Verification items for the finished model (mm, model axes). A direction names the side the tool comes from. Round coordinates to 2 decimals unless told otherwise and drop trailing zeros. Write each loop counter-clockwise with the first axis right and the second up, starting at its lowest first coordinate (ties: lowest second). Pieces come first, ordered by that corner, then holes. Notation, with made-up numbers: (18, 40) - (56, 40) arc R18 ccw to (56, 49) - close; hole circle Ø3 at (57.25, 68.25). An arc over 180 degrees is marked (long way). Answer as a JSON object with one key per item and string values.
Autodesk Inventor part; units mm, degrees
ref_plane "cut1_XY" through (13.4874, 7.874, 0) normal (1, 0, 0) x (0, 0, -1)
ref_plane "cut1_YZ" through (13.4874, 7.874, 0) normal (0, 0, -1) x (0, 1, 0)
ref_plane "cut1_ZX" through (13.4874, 7.874, 0) normal (0, 1, 0) x (1, 0, 0)
sketch "Sketch_1" plane through (0, 0, 0) normal (0, 0, 1) x (1, 0, 0)
  line L0 (13.4874, 0) -> (0, 0)
  line L1 (0, 0) -> (0, 8.9091)
  line L2 (0, 8.9091) -> (0.762, 9.671)
  line L3 (0.762, 9.671) -> (4.0386, 9.671)
  line L4 (4.0386, 9.671) -> (4.8006, 8.9091)
  line L5 (4.8006, 8.9091) -> (5.5626, 8.9091)
  line L6 (5.5626, 8.9091) -> (5.5626, 10.2235)
  line L7 (5.5626, 10.2235) -> (13.4874, 10.2235)
  line L8 (13.4874, 10.2235) -> (13.4874, 0)
  line L9 (13.4874, 0) -> (0, 0)
revolve "Revolution1" add sketch "Sketch_1" angle 360 about axis through (13.4874, 0, 0) along (1, 0, 0)
sketch "Sketch_6" plane through (0, 0, 0) normal (0, 0, 1) x (1, 0, 0)
  line L0 (13.4874, 0) -> (0, 0)
  line L1 (0, 0) -> (0, 4.3688)
  line L2 (0, 4.3688) -> (-1.5889, 4.3688)
  line L3 (-1.5889, 4.3688) -> (12.8524, 4.8197)
  line L4 (12.8524, 4.8197) -> (13.4874, 5.4547)
  line L5 (13.4874, 5.4547) -> (13.4874, 0)
  line L6 (13.4874, 0) -> (0, 0)
revolve "Revolution2" cut sketch "Sketch_6" angle 360 about axis through (13.4874, 0, 0) along (1, 0, 0)
thread "Thread1"
sketch "Sketch_5" plane through (13.4874, 0, 0) normal (1, 0, 0) x (0, 0, -1)
  line L0 (-40.894, -20.447) -> (40.894, -20.447)
  line L1 (40.894, -20.447) -> (40.894, 20.447)
  line L2 (40.894, 20.447) -> (-40.894, 20.447)
  line L3 (-40.894, 20.447) -> (-40.894, -20.447)
  line L4 (-20.447, -7.874) -> (20.447, -7.874)
  line L5 (20.447, -7.874) -> (20.447, 7.874)
  line L6 (20.447, 7.874) -> (-20.447, 7.874)
  line L7 (-20.447, 7.874) -> (-20.447, -7.874)
extrude "Extrusion1" cut sketch "Sketch_5" against normal blind 4.7752
sketch "Sketch_24" plane through (0, 0, 0) normal (0, 0, 1) x (1, 0, 0)
  line L0 (5.5626, 0) -> (4.8006, 0)
  line L1 (4.6479, 10.2235) -> (4.6479, 10.1393)
  line L2 (4.6479, 10.1393) -> (5.4401, 9.3472)
  arc A0 (5.4401, 9.1676) -> (5.4401, 9.3472) centre (5.3503, 9.2574) ccw
  line L3 (5.4401, 9.1676) -> (5.1816, 8.9091)
  line L4 (5.1816, 8.9091) -> (4.8006, 8.9091)
  line L5 (4.8006, 8.9091) -> (4.8006, 8.655)
  line L6 (4.8006, 8.655) -> (5.5626, 8.655)
  line L7 (5.5626, 8.655) -> (5.5626, 9.512)
  line L8 (5.5626, 9.512) -> (4.8511, 10.2235)
  line L9 (4.8511, 10.2235) -> (4.6479, 10.2235)
revolve "Revolution3" add sketch "Sketch_24" angle 360 about axis through (5.5626, 0, 0) along (1, 0, 0)
ref_plane "cut1_XY" through (13.4874, 7.874, 0) normal (1, 0, 0) x (0, 0, -1)
ref_plane "cut1_YZ" through (13.4874, 7.874, 0) normal (0, 0, -1) x (0, 1, 0)
ref_plane "cut1_ZX" through (13.4874, 7.874, 0) normal (0, 1, 0) x (1, 0, 0)
ref_plane "cut2_XY" through (13.4874, -7.874, 0) normal (1, 0, 0) x (0, 0, -1)
ref_plane "cut2_YZ" through (13.4874, -7.874, 0) normal (0, 0, -1) x (0, 1, 0)
ref_plane "cut2_ZX" through (13.4874, -7.874, 0) normal (0, 1, 0) x (1, 0, 0)
ref_plane "cutf1_XY" through (13.4874, 0, 0) normal (0, 0, 1) x (1, 0, 0)
ref_plane "cutf1_YZ" through (13.4874, 0, 0) normal (1, 0, 0) x (0, 1, 0)
ref_plane "cutf1_ZX" through (13.4874, 0, 0) normal (0, 1, 0) x (0, 0, 1)
ref_plane "cutf2_XY" through (8.7122, 0, 0) normal (0, 0, 1) x (1, 0, 0)
ref_plane "cutf2_YZ" through (8.7122, 0, 0) normal (1, 0, 0) x (0, 1, 0)
ref_plane "cutf2_ZX" through (8.7122, 0, 0) normal (0, 1, 0) x (0, 0, 1)
ref_plane "lovra_XY" through (13.4874, 0, 0) normal (1, 0, 0) x (0, 1, 0)
ref_plane "lovra_YZ" through (13.4874, 0, 0) normal (0, 1, 0) x (0, 0, 1)
ref_plane "lovra_ZX" through (13.4874, 0, 0) normal (0, 0, 1) x (1, 0, 0)
ref_plane "lovra1_XY" through (8.7122, 0, 0) normal (1, 0, 0) x (0, 0, -1)
ref_plane "lovra1_YZ" through (8.7122, 0, 0) normal (0, 0, -1) x (0, 1, 0)
ref_plane "lovra1_ZX" through (8.7122, 0, 0) normal (0, 1, 0) x (1, 0, 0)
ref_plane "lovra2_XY" through (8.7122, 7.874, 0) normal (1, 0, 0) x (0, 0, -1)
ref_plane "lovra2_YZ" through (8.7122, 7.874, 0) normal (0, 0, -1) x (0, 1, 0)
ref_plane "lovra2_ZX" through (8.7122, 7.874, 0) normal (0, 1, 0) x (1, 0, 0)
ref_plane "lovra21_XY" through (0, 0, 5.2705) normal (1, 0, 0) x (0, 0, -1)
ref_plane "lovra21_YZ" through (0, 0, 5.2705) normal (0, 0, -1) x (0, 1, 0)
ref_plane "lovra21_ZX" through (0, 0, 5.2705) normal (0, 1, 0) x (1, 0, 0)
ref_plane "lovra22_XY" through (0, 0, -5.2705) normal (1, 0, 0) x (0, 0, -1)
ref_plane "lovra22_YZ" through (0, 0, -5.2705) normal (0, 0, -1) x (0, 1, 0)
ref_plane "lovra22_ZX" through (0, 0, -5.2705) normal (0, 1, 0) x (1, 0, 0)
ref_plane "lovra3_XY" through (8.7122, -7.874, 0) normal (1, 0, 0) x (0, 0, -1)
ref_plane "lovra3_YZ" through (8.7122, -7.874, 0) normal (0, 0, -1) x (0, 1, 0)
ref_plane "lovra3_ZX" through (8.7122, -7.874, 0) normal (0, 1, 0) x (1, 0, 0)
ref_plane "olen_XY" through (13.4874, 0, 0) normal (1, 0, 0) x (0, 0, -1)
ref_plane "olen_YZ" through (13.4874, 0, 0) normal (0, 0, -1) x (0, 1, 0)
ref_plane "olen_ZX" through (13.4874, 0, 0) normal (0, 1, 0) x (1, 0, 0)
ref_plane "to_mounting_bracket_XY" through (24.6126, 0, 0) normal (1, 0, 0) x (0, 0, -1)
ref_plane "to_mounting_bracket_YZ" through (24.6126, 0, 0) normal (0, 0, -1) x (0, 1, 0)
ref_plane "to_mounting_bracket_ZX" through (24.6126, 0, 0) normal (0, 1, 0) x (1, 0, 0)
ref_plane "to_nut_XY" through (0, 0, 0) normal (1, 0, 0) x (0, 0, -1)
ref_plane "to_nut_YZ" through (0, 0, 0) normal (0, 0, -1) x (0, 1, 0)
ref_plane "to_nut_ZX" through (0, 0, 0) normal (0, 1, 0) x (1, 0, 0)
ref_plane "to_pin_XY" through (33.3248, 0, 0) normal (0, 1, 0) x (1, 0, 0)
ref_plane "to_pin_YZ" through (33.3248, 0, 0) normal (1, 0, 0) x (0, 0, -1)
ref_plane "to_pin_ZX" through (33.3248, 0, 0) normal (0, 0, -1) x (0, 1, 0)
ref_plane "to_pin_1_XY" through (33.3248, 0, 0) normal (0, 0, 1) x (1, 0, 0)
ref_plane "to_pin_1_YZ" through (33.3248, 0, 0) normal (1, 0, 0) x (0, 1, 0)
ref_plane "to_pin_1_ZX" through (33.3248, 0, 0) normal (0, 1, 0) x (0, 0, 1)
ref_plane "to_pin_r_XY" through (33.3248, 0, 0) normal (0, 0, 1) x (1, 0, 0)
ref_plane "to_pin_r_YZ" through (33.3248, 0, 0) normal (1, 0, 0) x (0, 1, 0)
ref_plane "to_pin_r_ZX" through (33.3248, 0, 0) normal (0, 1, 0) x (0, 0, 1)
ref_plane "to_screw_XY" through (17.4752, 2.032, -6.0452) normal (0, 1, 0) x (1, 0, 0)
ref_plane "to_screw_YZ" through (17.4752, 2.032, -6.0452) normal (1, 0, 0) x (0, 0, -1)
ref_plane "to_screw_ZX" through (17.4752, 2.032, -6.0452) normal (0, 0, -1) x (0, 1, 0)
ref_plane "to_tube_XY" through (4.8006, 0, 0) normal (1, 0, 0) x (0, 0, -1)
ref_plane "to_tube_YZ" through (4.8006, 0, 0) normal (0, 0, -1) x (0, 1, 0)
ref_plane "to_tube_ZX" through (4.8006, 0, 0) normal (0, 1, 0) x (1, 0, 0)
properties part number "040000_rear_head"
Q1. Release check for a two-part mould opening along X. For faces 6 (the flat face through (0, -2.1, 4.1)), 7 (the flat face through (5.563, 7, -7)), 8 (the flat face through (13.487, -5.4, 2.4)), 9 (the flat face through (11, 7.874, 0)) record: released by +X, released by -X, zero draft, split by the parting line, or undercut.
Geometry check:
{"face 6": "released by -X", "face 7": "undercut", "face 8": "released by +X", "face 9": "zero draft"}
Q2. Section check C-C, the plane x = 8. Record the cut outline in (y, z), then the cut area to 3 significant figures.
Geometry check:
{"outline": "circle Ø20.45 at (0, 0); hole circle Ø9.34 at (0, 0)", "area": "260 mm2"}
Q3. Gauge pin test, flat ends, axial feed: P1, Ø4, axis at x = 10, z = 3, coming from the +Y side; P2, Ø0.7, axis at y = -9, z = -1, coming from the +X side; P3, Ø1, axis at x = 4, y = 8, coming from the -Z side. Record the tip position at first contact, or that the pin passes through.
Geometry check:
{"P1": "stops at y = 10.12", "P2": "stops at x = 8.71", "P3": "stops at z = -6.11"}
Q4. Section check B-B, the plane x = 6. Record the cut outline in (y, z).
Geometry check:
{"outline": "circle Ø20.45 at (0, 0); hole circle Ø9.21 at (0, 0)"}
Q5. Set-up check for faces 1 (the cylindrical face through (4.994, -1.931, -8.697)), 2 (the cylindrical face through (2.42, -2.1, -9.44)), 3 (the flat face through (8.712, -9, 0)), 4 (the flat face through (8.712, 9, 0)), 5 (the cylindrical face through (8.7, -1.331, 10.137)): record each of +Z, -Z, +X, -X, +Y, -Y from which the full face is reachable in a straight line by a thin tool's end or side.
Geometry check:
{"face 1": "none", "face 2": "-X", "face 3": "+Z, -Z, +X, -Y", "face 4": "+Z, -Z, +X, +Y", "face 5": "+X, -X"}
Q6. Material ranges on line 1 along Z through (x, y) = (5, -0.75); line 2 along Z through (x, y) = (3.25, 2.5); line 3 along Z through (x, y) = (11.75, 3.75), recorded low to high. Write a range as [from, to].
Geometry check:
{"line 1": "z = [-10.05, -9.76], [-8.88, -4.51], [4.51, 8.88], [9.76, 10.05]", "line 2": "z = [-9.34, -3.77], [3.77, 9.34]", "line 3": "z = [-9.51, -2.97], [2.97, 9.51]"}
